Work out the finished part from the listing and answer in its coordinate system (mm). Face numbers are marked on the shaded views. A direction names the side the tool comes from. Give positions to 0.01 mm unless a question says otherwise; leave off trailing zeros. Order: outer loops, then holes, each group sorted by start corner. A loop starts at its lowest first (then second) coordinate and runs counter-clockwise, first axis right, second up. Notation, with made-up numbers: (21.25, 76.25) -> (68.25, 76.25) arc R16 cw to (68.25, 91.25) -> close; hole circle Ø7 at (63, -34). An arc over 180 degrees is marked (long way). Answer as CSV lines item,"result". Start each with the question number.
1. Find the intervals of material crossed by L1, parallel to X at y = -0.5, z = 48; L2, parallel to X at y = -26, z = 12.5; L3, parallel to Z at x = -31, y = -17, in increasing order.
2. A cutting plane is placed at B-B (x = -18). Give the vertices of the cut face in (y, z), then the cut area to 3 significant figures.
3. For a pull along X with two mould halves and no side action, classify the marked faces 1, 2 and 3 as released by +X, released by -X, zero draft, split by the parting line, or undercut.
4. A cutting plane is placed at D-D (z = 38.5). Give the vertices of the cut face in (x, y).
5. For the marked faces 4 and 5, determine the directions among +Z, -Z, +X, -X, +Y, -Y from which every point of the face is accessible in a straight line to the end or side of a thin tool.
6. A cutting plane is placed at A-A (z = 24). Give the vertices of the cut face in (x, y).
7. Flat-ended cylindrical pins translate along their axes: pin 1 (2 mm diameter, centred on x = -4.5, y = -23.5, fed in from -Z); pin 2 (3.5 mm diameter, centred on x = -9, y = 15.59, fed in from -Z); pin 3 (3.5 mm diameter, centred on x = -32.5, z = 45, fed in from -Y); pin 4 (1.5 mm diameter, centred on x = 16, y = -9, fed in from +Z). Find the tip coordinate at first contact, or state that the pin passes through.
8. A cutting plane is placed at C-C (y = 23). Give the vertices of the cut face in (x, z), then the cut area to 3 significant figures.
from build123d import *
from build123d.topology import SkipClean

# Parameters (mm, degrees)
SKETCH3_R           = 40
SKETCH3_R_2         = 2.05
SKETCH3_R_3         = 10
BOSS_EXTRUDE1_DEPTH = 5
BOSS_EXTRUDE2_DEPTH = 41
SKETCH5_W           = 112.43258682
SKETCH5_H           = 89.925085182
CUT_EXTRUDE1_DEPTH  = 100
CUT_EXTRUDE2_START  = 5
CUT_EXTRUDE2_DEPTH  = 82
CUT_EXTRUDE3_START  = -22
SKETCH7_R           = 11.1
CUT_EXTRUDE3_DEPTH  = 7.1
BOSS_EXTRUDE3_START = -22
SKETCH9_W           = 6.75
SKETCH9_H           = 25
BOSS_EXTRUDE3_DEPTH = 12.5
SKETCH8_R           = 2.05
SKETCH8_W           = 41
SKETCH8_H           = 21
CUT_EXTRUDE5_DEPTH  = 50
CHAMFER1_SIZE       = 5
CHAMFER2_SIZE       = 6
CUT_EXTRUDE6_START  = 33
SKETCH10_R          = 11.1
CUT_EXTRUDE6_DEPTH  = 7
CUT_EXTRUDE7_START  = -22
SKETCH11_W          = 55
SKETCH11_H          = 26
CUT_EXTRUDE7_DEPTH  = 6.5


with BuildPart() as part:
    # Sketch3 → Boss-Extrude1 (new body)
    with BuildSketch(Plane(origin=(0, 0, 0), x_dir=(0, 1, 0), z_dir=(0, 0, 1))):
        with Locations(Location((0, 0, 0), (0, 0, 270))):
            Circle(SKETCH3_R)
        with Locations(Location((0, 18, 0), (0, 0, 270))):
            Circle(SKETCH3_R_2, mode=Mode.SUBTRACT)
        with Locations(Location((15.588457268, 9, 0), (0, 0, 270))):
            Circle(SKETCH3_R_2, mode=Mode.SUBTRACT)
        with Locations(Location((15.588457268, -9, 0), (0, 0, 270))):
            Circle(SKETCH3_R_2, mode=Mode.SUBTRACT)
        with Locations(Location((0, -18, 0), (0, 0, 270))):
            Circle(SKETCH3_R_2, mode=Mode.SUBTRACT)
        with Locations(Location((-15.588457268, -9, 0), (0, 0, 270))):
            Circle(SKETCH3_R_2, mode=Mode.SUBTRACT)
        with Locations(Location((-15.588457268, 9, 0), (0, 0, 270))):
            Circle(SKETCH3_R_2, mode=Mode.SUBTRACT)
        with Locations(Location((0, 0, 0), (0, 0, 270))):
            Circle(SKETCH3_R_3, mode=Mode.SUBTRACT)
    extrude(amount=BOSS_EXTRUDE1_DEPTH)

    # Sketch4 → Boss-Extrude2 (add, symmetric)
    with BuildSketch(Plane.YZ):
        with BuildLine():
            Line((-40, 5), (-28.187426516, 59.125004254))
            ThreePointArc((-28.187426516, 59.125004254), (5.55857639, 86.659175658), (40, 60))
            Line((40, 60), (40, 5))
            Line((40, 5), (-40, 5))
        make_face()
    extrude(amount=BOSS_EXTRUDE2_DEPTH, both=True)

    # Sketch5 → Cut-Extrude1 (cut)
    with SkipClean():  # the faces are left unmerged after this step: merging them gives an invalid solid
        with BuildSketch(Plane(origin=(0, 0, 0), x_dir=(0, 1, 0), z_dir=(0, 0, 1))):
            Rectangle(SKETCH5_W, SKETCH5_H)
            with BuildLine():
                Line((-20.24228248, 34.5), (20.24228248, 34.5))
                ThreePointArc((20.24228248, 34.5), (0, -40), (-20.24228248, 34.5))
            make_face(mode=Mode.SUBTRACT)
        extrude(amount=CUT_EXTRUDE1_DEPTH, mode=Mode.SUBTRACT)
    add(part.part.scale(1), mode=Mode.REPLACE)  # the faces are merged on a copy

    # Sketch6 → Cut-Extrude2 (cut)
    with BuildSketch(Plane(origin=(0, 0, 0), x_dir=(0, 1, 0), z_dir=(0, 0, 1)).offset(CUT_EXTRUDE2_START)):
        with BuildLine():
            Line((-13.85765721, -26), (13.85765721, -26))
            Line((13.85765721, -26), (30.397368307, -26))
            ThreePointArc((30.397368307, -26), (39.921625117, -2.502768077), (33.406586177, 22))
            Line((33.406586177, 22), (-33.406586177, 22))
            ThreePointArc((-33.406586177, 22), (-39.921625117, -2.502768077), (-30.397368307, -26))
            Line((-30.397368307, -26), (-13.85765721, -26))
        make_face()
        with BuildLine():
            Line((-20.24228248, 34.5), (20.24228248, 34.5))
            ThreePointArc((20.24228248, 34.5), (0, 40), (-20.24228248, 34.5))
        make_face()
    extrude(amount=CUT_EXTRUDE2_DEPTH, mode=Mode.SUBTRACT)

    # Sketch7 → Cut-Extrude3 (cut)
    with BuildSketch(Plane.YZ.offset(CUT_EXTRUDE3_START)):
        with Locations(Location((-3, 29, 0), (0, 0, 270))):
            Circle(SKETCH7_R)
    extrude(amount=-CUT_EXTRUDE3_DEPTH, mode=Mode.SUBTRACT)

    # Sketch9 → Boss-Extrude3 (add)
    with BuildSketch(Plane.YZ.offset(BOSS_EXTRUDE3_START)):
        with Locations((30, 59.998090913)):
            Rectangle(SKETCH9_W, SKETCH9_H)
    extrude(amount=-BOSS_EXTRUDE3_DEPTH)

    # Sketch8 → Cut-Extrude5 (cut)
    with BuildSketch(Plane.YZ):
        with Locations(Location((-17.5, 65.15, 0), (0, 0, 270))):
            Circle(SKETCH8_R)
        with Locations(Location((-17.5, 54.95, 0), (0, 0, 270))):
            Circle(SKETCH8_R)
        with Locations((31.5, 54.95)):
            Circle(SKETCH8_R)
        with Locations((31.5, 65.15)):
            Circle(SKETCH8_R)
        with Locations((7, 60.05)):
            Rectangle(SKETCH8_W, SKETCH8_H)
    extrude(amount=-CUT_EXTRUDE5_DEPTH, mode=Mode.SUBTRACT)

    # Chamfer1
    # the kernel refuses this chamfer: 5 mm, written as the material it adds along each edge
    with BuildSketch(Plane(origin=(0, 0, 72.498090913), x_dir=(-0.9183651186253444, 0.39573413915437844, 0), z_dir=(-0.39573413915437844, -0.9183651186253444, 0))) as chamfer1_piece_1_section:
        Polygon((40, -CHAMFER1_SIZE), (40 + CHAMFER1_SIZE, 0), (40, 0), align=None)
    chamfer1_piece_1 = revolve(axis=Axis((0, 0, 72.498090913), (0, 0, -1)), revolution_arc=51.657569858, mode=Mode.PRIVATE)
    chamfer1_piece_1 = split(chamfer1_piece_1, bisect_by=Plane(origin=(-34.5, 29.836622418, 73.971077773), z_dir=(1, 0, 0)), keep=Keep.TOP, mode=Mode.PRIVATE)
    chamfer1_piece_1 = split(chamfer1_piece_1, bisect_by=Plane(origin=(-22, 29.836622418, 73.971077773), z_dir=(-1, 0, 0)), keep=Keep.TOP, mode=Mode.PRIVATE)
    chamfer1_piece_1 = chamfer1_piece_1 & Plane(origin=(-28.977022362, 6.007666956, 51.662056953), x_dir=(0, -0.9770026706356161, 0.21322706575590716), z_dir=(1, 0, 0)) * Cylinder(35, 180, mode=Mode.PRIVATE)
    chamfer1_piece_1 = split(chamfer1_piece_1, bisect_by=Plane(origin=(-28.977022362, 33.375, 73.971077773), z_dir=(0, -1, 0)), keep=Keep.TOP, mode=Mode.PRIVATE)
    chamfer1_piece_1 = split(chamfer1_piece_1, bisect_by=Plane(origin=(-28.977022362, 26.625, 73.971077773), z_dir=(0, 1, 0)), keep=Keep.TOP, mode=Mode.PRIVATE)
    add(chamfer1_piece_1)
    with BuildSketch(Plane(origin=(0, 0, 47.498090913), x_dir=(-0.9183651186253442, 0.39573413915437894, 0), z_dir=(-0.39573413915437894, -0.9183651186253442, 0))) as chamfer1_piece_2_section:
        Polygon((40, CHAMFER1_SIZE), (40 + CHAMFER1_SIZE, 0), (40, 0), align=None)
    chamfer1_piece_2 = revolve(axis=Axis((0, 0, 47.498090913), (0, 0, -1)), revolution_arc=51.657569858, mode=Mode.PRIVATE)
    chamfer1_piece_2 = split(chamfer1_piece_2, bisect_by=Plane(origin=(-34.5, 30.172032739, 45.811526919), z_dir=(1, 0, 0)), keep=Keep.TOP, mode=Mode.PRIVATE)
    chamfer1_piece_2 = split(chamfer1_piece_2, bisect_by=Plane(origin=(-28.439026237, 26.625, 45.811526919), z_dir=(0, 1, 0)), keep=Keep.TOP, mode=Mode.PRIVATE)
    chamfer1_piece_2 = split(chamfer1_piece_2, bisect_by=Plane(origin=(-28.439026237, 33.375, 45.811526919), z_dir=(0, -1, 0)), keep=Keep.TOP, mode=Mode.PRIVATE)
    chamfer1_piece_2 = split(chamfer1_piece_2, bisect_by=Plane(origin=(-22, 30.172032739, 45.811526919), z_dir=(-1, 0, 0)), keep=Keep.TOP, mode=Mode.PRIVATE)
    add(chamfer1_piece_2)

    # Chamfer2
    # the kernel refuses this chamfer: 6 mm, written as the material it adds along each edge
    with BuildSketch(Plane(origin=(26, -45.827466235, 5), x_dir=(-0.9996219169112969, 0, -0.027495876610586355), z_dir=(0, 1, 0))) as chamfer2_piece_1_section:
        Polygon((CHAMFER2_SIZE * 0.999621916911, CHAMFER2_SIZE * 0.0274958766106), (-CHAMFER2_SIZE * 0.0274958766106, CHAMFER2_SIZE * 0.999621916911), (0, 0), align=None)
    chamfer2_piece_1 = extrude(amount=91.65493247, mode=Mode.PRIVATE)
    chamfer2_piece_1 = chamfer2_piece_1 & Plane(origin=(0, 0, 6.950735371), x_dir=(1, 0, 0), z_dir=(0, 0, -1)) * Cylinder(40, 208, mode=Mode.PRIVATE)
    chamfer2_piece_1 = chamfer2_piece_1 - Plane(origin=(18, 0, 6.950735371), x_dir=(1, 0, 0), z_dir=(0, 0, -1)) * Cylinder(2.05, 208, mode=Mode.PRIVATE)
    add(chamfer2_piece_1)
    with BuildSketch(Plane(origin=(-22, 48.836684105, 5), x_dir=(0.9996219169112969, 0, -0.027495876610586348), z_dir=(0, -1, 0))) as chamfer2_piece_2_section:
        Polygon((CHAMFER2_SIZE * 0.999621916911, CHAMFER2_SIZE * 0.0274958766106), (-CHAMFER2_SIZE * 0.0274958766106, CHAMFER2_SIZE * 0.999621916911), (0, 0), align=None)
    chamfer2_piece_2 = extrude(amount=97.67336821, mode=Mode.PRIVATE)
    chamfer2_piece_2 = chamfer2_piece_2 & Plane(origin=(0, 0, 5.808875482), x_dir=(1, 0, 0), z_dir=(0, 0, -1)) * Cylinder(40, 220, mode=Mode.PRIVATE)
    chamfer2_piece_2 = chamfer2_piece_2 - Plane(origin=(-18, 0, 5.808875482), x_dir=(1, 0, 0), z_dir=(0, 0, -1)) * Cylinder(2.05, 220, mode=Mode.PRIVATE)
    add(chamfer2_piece_2)

    # Sketch10 → Cut-Extrude6 (cut)
    with BuildSketch(Plane.YZ.offset(CUT_EXTRUDE6_START)):
        with Locations(Location((-3, 29, 0), (0, 0, 270))):
            Circle(SKETCH10_R)
    extrude(amount=-CUT_EXTRUDE6_DEPTH, mode=Mode.SUBTRACT)

    # Sketch11 → Cut-Extrude7 (cut)
    with BuildSketch(Plane.YZ.offset(CUT_EXTRUDE7_START)):
        with Locations((7, 60.05)):
            Rectangle(SKETCH11_W, SKETCH11_H)
    extrude(amount=-CUT_EXTRUDE7_DEPTH, mode=Mode.SUBTRACT)


solid = part.part
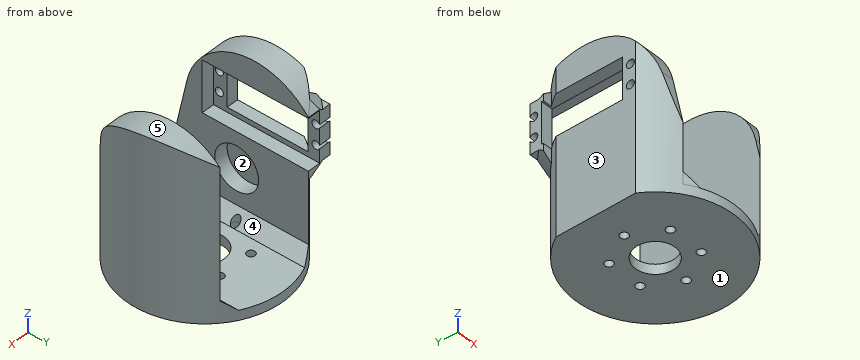
Answer sheet:
1,L1,"x = -34.5 to -28.5, 26 to 40"
1,L2,"x = -30.4 to -22, 26 to 30.4"
1,L3,"z = 0 to 52.96, 56.94 to 63.16, 67.14 to 78.04"
2,outline,"(-35.72, 0) -> (-2.05, 0) -> (-2.05, 7) -> (-35.72, 7) -> close; (2.05, 0) -> (35.72, 0) -> (35.72, 7) -> (2.05, 7) -> close"
2,area,"471 mm^2"
3,face 1,"zero draft"
3,face 2,"undercut"
3,face 3,"released by -X"
4,outline,"(-34.5, -20.24) arc R40 ccw to (-23.05, -32.69) -> (-22, -32.69) -> (-22, -8.74) -> (-29.1, -8.74) -> (-29.1, 2.74) -> (-22, 2.74) -> (-22, 33.41) arc R40 ccw to (-34.5, 20.24) -> close; (26, -30.4) arc R40 ccw to (26, 30.4) -> (26, 2.74) -> (33, 2.74) -> (33, -8.74) -> (26, -8.74) -> close"
5,face 4,"+Z, +Y, -Y"
5,face 5,"+Z, +X, -X"
6,outline,"(-34.5, -20.24) arc R40 ccw to (-22, -33.41) -> (-22, -12.91) -> (-29.1, -12.91) -> (-29.1, 6.91) -> (-22, 6.91) -> (-22, 33.41) arc R40 ccw to (-34.5, 20.24) -> close; (26, -30.4) arc R40 ccw to (26, 30.4) -> (26, 6.91) -> (33, 6.91) -> (33, -12.91) -> (26, -12.91) -> close"
7,pin 1,"stops at z = 0"
7,pin 2,"passes through"
7,pin 3,"stops at y = -25.58"
7,pin 4,"stops at z = 5"
8,outline,"(-32.73, 0) -> (32.73, 0) -> (32.73, 82.26) -> (26, 82.26) -> (26, 11) -> (20, 5) -> (-16, 5) -> (-22, 11) -> (-22, 47.05) -> (-28.5, 47.05) -> (-28.5, 49.55) -> (-32.73, 49.55) -> close; (-32.73, 70.55) -> (-28.5, 70.55) -> (-28.5, 73.05) -> (-22, 73.05) -> (-22, 82.26) -> (-32.73, 82.26) -> close"
8,area,"1,450 mm^2"
